```python
from build123d import *

# Parameters (mm, degrees)
SKETCH_R        = 1.5
PAD_DEPTH       = 22
SKETCH001_R     = 12
SKETCH001_R_2   = 1.65
POCKET_DEPTH    = 3.001
CHAMFER_SIZE    = 0.5
CHAMFER001_SIZE = 4
SKETCH002_R     = 3
SKETCH002_R_2   = 1.8
PAD001_DEPTH    = 1
CHAMFER002_SIZE = 0.5


with BuildPart() as part:
    # Sketch → Pad (new body, symmetric)
    with BuildSketch(Plane.XZ):
        with BuildLine():
            ThreePointArc((5, 5.000025), (-3.535543, 8.535525), (0, 0))
            Line((0, 0), (55, 0))
            Line((55, 0), (55, 3))
            Line((55, 3), (5, 3))
            Line((5, 3), (5, 5.000025))
        make_face()
        with Locations((0, 5)):
            Circle(SKETCH_R, mode=Mode.SUBTRACT)
    extrude(amount=PAD_DEPTH, both=True)

    # Sketch001 → Pocket (cut, through all)
    with BuildSketch(Plane(origin=(0, 0, 3), x_dir=(-1, 0, 0), z_dir=(0, 0, 1))):
        with Locations((-33.5, 0)):
            Circle(SKETCH001_R)
        with Locations((-49, 15.5)):
            Circle(SKETCH001_R_2)
        with Locations((-18, 15.5)):
            Circle(SKETCH001_R_2)
        with Locations((-18, -15.5)):
            Circle(SKETCH001_R_2)
        with Locations((-49, -15.5)):
            Circle(SKETCH001_R_2)
    extrude(amount=-POCKET_DEPTH, mode=Mode.SUBTRACT)

    # Chamfer
    chamfer_edges = [part.edges().sort_by_distance(p)[0] for p in [
        (-1.5, -22, 5),
        (-1.5, 22, 5),
    ]]
    chamfer(chamfer_edges, length=CHAMFER_SIZE)

    # Chamfer001
    chamfer001_edges = [part.edges().sort_by_distance(p)[0] for p in [
        (55, 22, 1.5),
        (55, -22, 1.5),
    ]]
    chamfer(chamfer001_edges, length=CHAMFER001_SIZE)

    # Sketch002 → Pad001 (new body)
    with BuildSketch(Plane(origin=(0, 0, 0), x_dir=(1, 0, 0), z_dir=(0, 0, -1))):
        with Locations((49, -15.5)):
            Circle(SKETCH002_R)
        with Locations((49, -15.5)):
            Circle(SKETCH002_R_2, mode=Mode.SUBTRACT)
        with Locations((18, 15.5)):
            Circle(SKETCH002_R)
        with Locations((18, 15.5)):
            Circle(SKETCH002_R_2, mode=Mode.SUBTRACT)
    extrude(amount=PAD001_DEPTH)

    # Chamfer002
    chamfer002_edges = [part.edges().sort_by_distance(p)[0] for p in [
        (46, 15.5, -1),
        (15, -15.5, -1),
    ]]
    chamfer(chamfer002_edges, length=CHAMFER002_SIZE)


solid = part.part
```
Part model, mm, in its own coordinate system. A direction names the side the tool comes from. Coordinates: 2 decimals unless noted, no trailing zeros. Loops run counter-clockwise (first coordinate to the right, second up) from the corner with the lowest first, then second, coordinate; pieces in that order, holes last. Notation, with made-up numbers: (48, 80) - (76, 80) arc R29 cw to (76, 114) - close; hole circle Ø2 at (-27, 27.5). An arc over 180 degrees is marked (long way). Write item = value, one per line. Start each with the question number.
Item 1: 3-axis set-ups, long thin cutter, end or side, ignore diameter. For faces 1 (the cylindrical face through (46.6, 17.3, -0.2)), 2 (the cylindrical face through (50.65, 15.43, 1.52)), 3 (the flat face through (19, 0, 3)): which of +Z, -Z, +X, -X, +Y, -Y reach the whole face in a straight line?
Item 2: Cut at A-A, the plane y = 15.5. Give the cut face in (x, z).
Item 3: Cut at D-D, the plane x = 18. Give the cut face in (y, z).
Item 4: Cut at B-B, the plane x = 33.5. Give the cut face in (y, z).
Item 5: Cut at C-C, the plane y = -6.5. Give the cut face in (x, z), and give its area (3 significant figures).
Item 6: Wall check: L1, parallel to Y at x = 18, z = 2.45; L2, parallel to X at y = -15.5, z = 1.4; L3, parallel to Z at x = 44, y = -16. Give the ranges that are in metal, low to high. Write a range as from..to.
Item 7: Flat gauge pins, fed straight in: pin 1 Ø22 at (x, y) = (17.5, 7.5) entering from -Z; pin 2 Ø13 at (x, y) = (23.5, 4) entering from +Z; pin 3 Ø0.6 at (y, z) = (3.5, 3.5) entering from +X. Where does each tip first touch, or does it go through?
The answers:
q1.face_1 = -Z
q1.face_2 = +Z, -Z
q1.face_3 = +Z, +X, +Y, -Y
q2.outline = (0, 0) - (16.35, 0) - (16.35, 3) - (5, 3) - (5, 5) arc R5 ccw (long way) to start; (19.65, 0) - (46, 0) - (46, -0.5) - (46.5, -1) - (47.2, -1) - (47.2, 0) - (47.35, 0) - (47.35, 3) - (19.65, 3) - close; (50.65, 0) - (50.8, 0) - (50.8, -1) - (51.5, -1) - (52, -0.5) - (52, 0) - (55, 0) - (55, 3) - (50.65, 3) - close; hole circle Ø3 at (0, 5)
q3.outline = (-22, 0) - (-18.5, 0) - (-18.5, -0.5) - (-18, -1) - (-17.3, -1) - (-17.3, 0) - (-17.15, 0) - (-17.15, 3) - (-22, 3) - close; (-13.85, 0) - (-13.7, 0) - (-13.7, -1) - (-13, -1) - (-12.5, -0.5) - (-12.5, 0) - (13.85, 0) - (13.85, 3) - (-13.85, 3) - close; (17.15, 0) - (22, 0) - (22, 3) - (17.15, 3) - close
q4.outline = (-22, 0) - (-12, 0) - (-12, 3) - (-22, 3) - close; (12, 0) - (22, 0) - (22, 3) - (12, 3) - close
q5.outline = (0, 0) - (23.41, 0) - (23.41, 3) - (5, 3) - (5, 5) arc R5 ccw (long way) to start; (43.59, 0) - (55, 0) - (55, 3) - (43.59, 3) - close; hole circle Ø3 at (0, 5)
q5.area = 166 mm2
q6.L1 = -22..-17.15, -13.85..13.85, 17.15..22
q6.L2 = -3.47..16.35, 19.65..47.35, 50.65..55
q6.L3 = 0..3
q7.pin_1 = 0
q7.pin_2 = 3
q7.pin_3 = 5
